```python
from build123d import *

# Parameters (mm, degrees)
SKETCH1_W           = 14.7
SKETCH1_H           = 4.8
BOSS_EXTRUDE1_DEPTH = 3.175
BOSS_EXTRUDE2_DEPTH = 5.461


with BuildPart() as part:
    # Sketch1 → Boss-Extrude1 (new body)
    with BuildSketch(Plane(origin=(0, 0, 0), x_dir=(1, 0, 0), z_dir=(0, 1, 0))):
        Rectangle(SKETCH1_W, SKETCH1_H)
    extrude(amount=BOSS_EXTRUDE1_DEPTH)

    # Sketch2 → Boss-Extrude2 (add)
    with BuildSketch(Plane(origin=(0, 3.175, 0), x_dir=(1, 0, 0), z_dir=(0, 1, 0))):
        with BuildLine():
            Line((-4.032, 1.032), (-1.048, 1.032))
            ThreePointArc((-1.048, 1.032), (-0.688789755, 0.883210245), (-0.54, 0.524))
            Line((-0.54, 0.524), (-0.54, 0))
            ThreePointArc((-0.54, 0), (-1.413, -0.873), (-2.286, 0))
            Line((-2.286, 0), (-2.159, 0))
            ThreePointArc((-2.159, 0), (-1.413, -0.746), (-0.667, 0))
            Line((-0.667, 0), (-0.667, 0.524))
            ThreePointArc((-0.667, 0.524), (-0.778592316, 0.793407684), (-1.048, 0.905))
            Line((-1.048, 0.905), (-4.032, 0.905))
            ThreePointArc((-4.032, 0.905), (-4.301407684, 0.793407684), (-4.413, 0.524))
            Line((-4.413, 0.524), (-4.413, 0))
            ThreePointArc((-4.413, 0), (-3.667, -0.746), (-2.921, 0))
            Line((-2.921, 0), (-2.794, 0))
            ThreePointArc((-2.794, 0), (-3.667, -0.873), (-4.54, 0))
            Line((-4.54, 0), (-4.54, 0.524))
            ThreePointArc((-4.54, 0.524), (-4.391210245, 0.883210245), (-4.032, 1.032))
        make_face()
        with BuildLine():
            Line((4.54, 0.524), (4.54, 0))
            ThreePointArc((4.54, 0), (3.667, -0.873), (2.794, 0))
            Line((2.794, 0), (2.921, 0))
            ThreePointArc((2.921, 0), (3.667, -0.746), (4.413, 0))
            Line((4.413, 0), (4.413, 0.524))
            ThreePointArc((4.413, 0.524), (4.301407684, 0.793407684), (4.032, 0.905))
            Line((4.032, 0.905), (1.048, 0.905))
            ThreePointArc((1.048, 0.905), (0.778592316, 0.793407684), (0.667, 0.524))
            Line((0.667, 0.524), (0.667, 0))
            ThreePointArc((0.667, 0), (1.413, -0.746), (2.159, 0))
            Line((2.159, 0), (2.286, 0))
            ThreePointArc((2.286, 0), (1.413, -0.873), (0.54, 0))
            Line((0.54, 0), (0.54, 0.524))
            ThreePointArc((0.54, 0.524), (0.688789755, 0.883210245), (1.048, 1.032))
            Line((1.048, 1.032), (4.032, 1.032))
            ThreePointArc((4.032, 1.032), (4.391210245, 0.883210245), (4.54, 0.524))
        make_face()
    extrude(amount=BOSS_EXTRUDE2_DEPTH)


solid = part.part
```
CAD build for the part. Positions are in the model's coordinates, mm. Give positions to 0.01 mm unless a question says otherwise; leave off trailing zeros. Order: outer loops, then holes, each group sorted by start corner. A loop starts at its lowest first (then second) coordinate and runs counter-clockwise, first axis right, second up.
(1) Saw through at C-C, the plane x = 5. Give the cut face in (y, z) (3 decimals).
(2) Saw through at A-A, the plane x = -2.5. Give the cut face in (y, z) (3 decimals), then the cut area to 3 significant figures.
(3) Flat gauge pins, fed straight in: pin 1 (3.5 mm diameter, centred on x = 3, y = 7, fed in from -Z); pin 2 (0.9 mm diameter, centred on x = 2, y = 6, fed in from +Z); pin 3 (0.6 mm diameter, centred on y = 5.5, z = 0, fed in from -X). Where does each tip first touch, or does it go through?
(4) Mould opens along X. For faces 1 (the flat face through (0, 3.175, 0)), 2 (the flat face through (7.35, 2, 0)), 3 (the flat face through (-7.35, 2, 0)) say: released by +X, released by -X, zero draft, split by the parting line, or undercut.
(5) Saw through at B-B, the plane z = -0.75. Give the cut face in (x, y) (3 decimals).
(6) Drill centre lines: L1, parallel to X at y = 3.25, z = -0.85; L2, parallel to Y at x = 0, z = 2.05 (3 decimals); L3, parallel to Z at x = 0.75, y = 5. Where is each one in solid material? Low to high.
Results found:
1. outline: (0, -2.4) - (3.175, -2.4) - (3.175, 2.4) - (0, 2.4) - close
2. outline: (0, -2.4) - (3.175, -2.4) - (3.175, -1.032) - (8.636, -1.032) - (8.636, -0.905) - (3.175, -0.905) - (3.175, 2.4) - (0, 2.4) - close
2. area: 15.9 mm2
3. pin 1: stops at z = -1.03
3. pin 2: stops at z = 0.86
3. pin 3: stops at x = -4.54
4. face 1: undercut
4. face 2: released by +X
4. face 3: released by -X
5. outline: (-7.35, 0) - (7.35, 0) - (7.35, 3.175) - (4.487, 3.175) - (4.487, 8.636) - (4.339, 8.636) - (4.339, 3.175) - (0.741, 3.175) - (0.741, 8.636) - (0.593, 8.636) - (0.593, 3.175) - (-0.593, 3.175) - (-0.593, 8.636) - (-0.741, 8.636) - (-0.741, 3.175) - (-4.339, 3.175) - (-4.339, 8.636) - (-4.487, 8.636) - (-4.487, 3.175) - (-7.35, 3.175) - close
6. L1: x = -4.42 to -4.23, -0.85 to -0.66, 0.66 to 0.85, 4.23 to 4.42
6. L2: y = 0 to 3.175
6. L3: z = -0.94 to -0.76, 0.34 to 0.57
